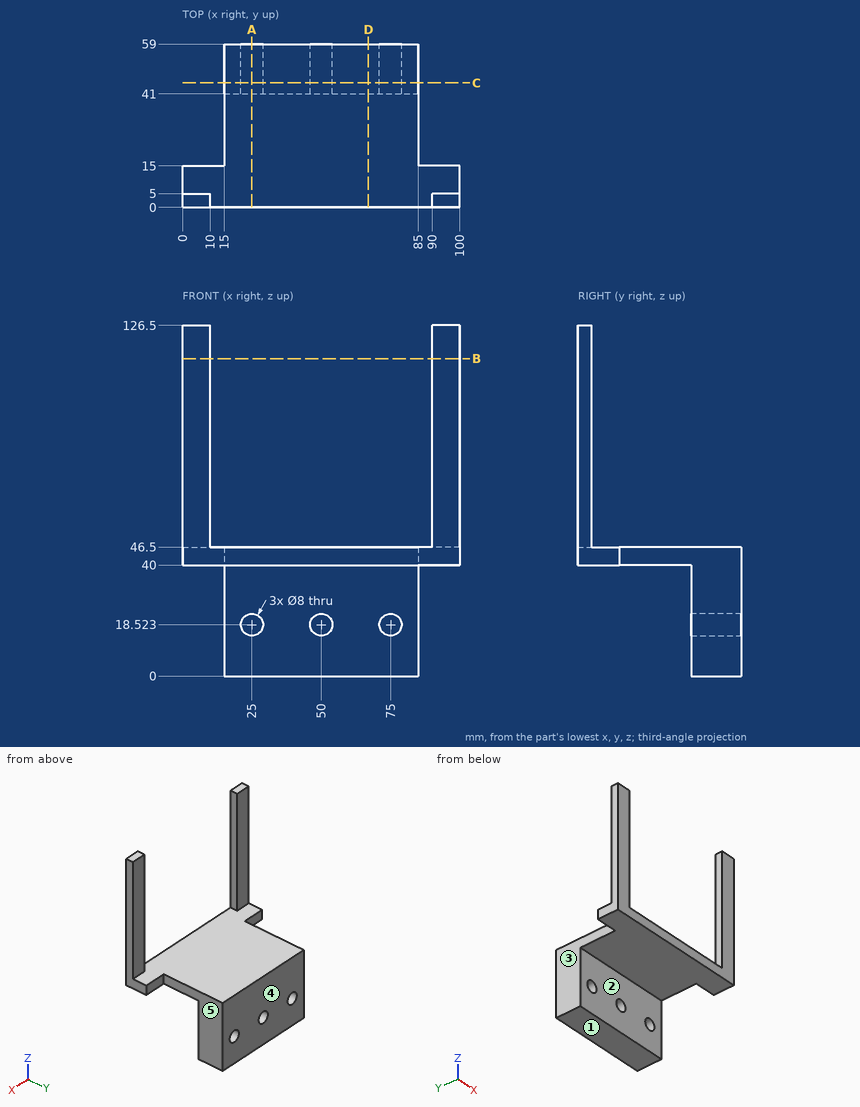
Study the drawing (mm; zero at the part's minimum x, y, z) and answer. A direction names the side the tool comes from. Coordinates: 2 decimals unless noted, no trailing zeros. Write each loop counter-clockwise with the first axis right and the second up, starting at its lowest first coordinate (ties: lowest second). Pieces come first, ordered by that corner, then holes.
Q1. Each of these flat-tipped pins is pushed along its axis until it touches: pin 1 Ø20.5 at (x, y) = (71, 12.5) entering from -Z; pin 2 Ø13 at (y, z) = (37.5, 13) entering from -X; pin 3 Ø3 at (x, z) = (92, 43) entering from +Y. Where does it stop, or does it pass through?
Q2. A cutting plane is placed at A-A, the plane x = 25. Give the vertices of the cut face in (y, z), then the cut area to 4 significant figures.
Q3. Which of the six approach directions +Z, -Z, +X, -X, +Y, -Y give full straight-line access (tool end or side, diameter ignored) to the marked faces 1, 2, 3, 4 and 5?
Q4. A cutting plane is placed at D-D, the plane x = 67. Give the vertices of the cut face in (y, z).
Q5. A cutting plane is placed at B-B, the plane z = 114.5. Give the vertices of the cut face in (x, y).
Q6. A cutting plane is placed at C-C, the plane y = 45. Give the vertices of the cut face in (x, z).
Q7. Find the intervals of material crossed by line 1 (X direction, y = 39, z = 43); line 2 (X direction, y = 4, z = 56.5); line 3 (Z direction, x = 77, y = 8), in increasing order.
Findings below:
1. pin 1: stops at z = 40
1. pin 2: stops at x = 15
1. pin 3: stops at y = 15
2. outline: (0, 40) - (41, 40) - (41, 22.52) - (59, 22.52) - (59, 46.5) - (0, 46.5) - close; (41, 0) - (59, 0) - (59, 14.52) - (41, 14.52) - close
2. area: 959.5 mm2
3. face 1: -Z, +X, -X, +Y, -Y
3. face 2: -Z, +X, -X, -Y
3. face 3: +Z, -Z, -X, +Y
3. face 4: +Z, -Z, +X, -X, +Y
3. face 5: +Z, -Z, +X, +Y
4. outline: (0, 40) - (41, 40) - (41, 0) - (59, 0) - (59, 46.5) - (0, 46.5) - close
5. outline: (0, 0) - (10, 0) - (10, 5) - (0, 5) - close; (90, 0) - (100, 0) - (100, 5) - (90, 5) - close
6. outline: (15, 0) - (85, 0) - (85, 46.5) - (15, 46.5) - close; hole circle Ø8 at (25, 18.52); hole circle Ø8 at (50, 18.52); hole circle Ø8 at (75, 18.52)
7. line 1: x = 15 to 85
7. line 2: x = 0 to 10, 90 to 100
7. line 3: z = 40 to 46.5
